```python
from build123d import *

# Parameters (mm, degrees)
F0_W          = 35
F0_H          = 89
F1_DEPTH      = 63
F2_T          = -4
F3_W          = 27
F3_H          = 7.0524177253
F4_DEPTH      = 4.3
F5_DEPTH      = 5.2
F7_DEPTH      = 12
F9_DEPTH      = 28.5
F8_W          = 16.7951798066
F8_H          = 6.5415552817
F10_DEPTH     = 15.6
F8_W_2        = 16.8639151379
F8_H_2        = 7.3436973616
F11_DEPTH     = 29.2
F8_W_3        = 16.7673844844
F8_H_3        = 8.8219475001
F12_DEPTH     = 48.1
F13_W         = 10
F13_H         = 10
F14_DEPTH     = 10
F15_W         = 10
F15_H         = 10
F16_DEPTH     = 10
F19_DEPTH     = 10
F20_DEPTH     = 10
F21_T1_DEPTH  = 97.5
F21_T3_DEPTH  = 27
F21_T8_DEPTH  = 94
F21_T13_DEPTH = 110
F21_T18_DEPTH = 110
F21_T23_DEPTH = 94
F21_T29_DEPTH = 97.5
F21_T35_DEPTH = 39.5
F21_T44_DEPTH = 39.5
F21_T50_DEPTH = 97.5


# Not quite as in the source:
# - a fillet or chamfer that OpenCascade refuses, or shapes differently, is made with other operations: its cross-section is extruded or revolved along the edge and cut away or added


with BuildPart() as f1:
    # F0 (on Top) → F1 (new body)
    with BuildSketch(Plane.XY):
        Rectangle(F0_W, F0_H)
    extrude(amount=F1_DEPTH)

    # F2
    f2_openings = [f1.faces().sort_by_distance(p)[0] for p in [
        (0, 0, 63),
    ]]
    offset(amount=F2_T, openings=f2_openings)

    # F3 (on face) → F4 (cut)
    with BuildSketch(Plane.XY.offset(4)):
        with Locations((0, 36.9737911373)):
            Rectangle(F3_W, F3_H)
    extrude(amount=-F4_DEPTH, mode=Mode.SUBTRACT)

    # F5 (cut): a face of the model
    f5_faces = [f1.faces().sort_by_distance(p)[0] for p in [
        (0, -40.5, 33.5),
    ]]
    extrude(f5_faces, amount=-F5_DEPTH, mode=Mode.SUBTRACT)

    # F7 (add): a face of the model
    f7_faces = [f1.faces().sort_by_distance(p)[0] for p in [
        (-16.5436527827, 0, 63),
    ]]
    extrude(f7_faces, amount=F7_DEPTH)

    # F6 (on face) → F9 (join)
    with BuildSketch(Plane(origin=(13.5, 0, 0), x_dir=(0, -1, 0), z_dir=(-1, 0, 0))):
        Polygon((44.5, 63), (-33.4475822747, 4), (-24.9599814415, 4), (44.5, 56.4169287682), align=None)
    extrude(amount=F9_DEPTH)

    # F8 (on face) → F10 (join)
    with BuildSketch(Plane.XY.offset(4)):
        with Locations((-0.0789728947, 8.664857829)):
            Rectangle(F8_W, F8_H)
    extrude(amount=F10_DEPTH)

    # F8 (on face) → F11 (join)
    with BuildSketch(Plane.XY.offset(4)):
        with Locations((-0.044605229, -10.0223287009)):
            Rectangle(F8_W_2, F8_H_2)
    extrude(amount=F11_DEPTH)

    # F8 (on face) → F12 (join)
    with BuildSketch(Plane.XY.offset(4)):
        with Locations((-0.0928705558, -34.9372858182)):
            Rectangle(F8_W_3, F8_H_3)
    extrude(amount=F12_DEPTH)

    # F13 (on face) → F14 (join)
    with BuildSketch(Plane.YZ.offset(17.5)):
        with Locations((-39.5, 70)):
            Rectangle(F13_W, F13_H)
        with Locations((39.5, 70)):
            Rectangle(F13_W, F13_H)
    extrude(amount=F14_DEPTH)

    # F15 (on face) → F16 (join)
    with BuildSketch(Plane(origin=(-17.5, 0, 0), x_dir=(0, -1, 0), z_dir=(-1, 0, 0))):
        with Locations((-39.5, 70)):
            Rectangle(F15_W, F15_H)
        with Locations((39.5, 70)):
            Rectangle(F15_W, F15_H)
    extrude(amount=F16_DEPTH)

    # F18 (on face) → F19 (cut)
    with BuildSketch(Plane.XZ.offset(44.5)):
        Polygon((-17.5, 65), (-27.5, 75), (-27.5, 65), align=None)
        Polygon((27.5, 75), (17.5, 65), (27.5, 65), align=None)
    extrude(amount=-F19_DEPTH, mode=Mode.SUBTRACT)

    # F17 (on face) → F20 (cut)
    with BuildSketch(Plane(origin=(0, 44.5, 0), x_dir=(-1, 0, 0), z_dir=(0, 1, 0))):
        Polygon((-17.5, 65), (-27.5, 75), (-27.5, 65), align=None)
        Polygon((27.5, 65), (27.5, 75), (17.5, 65), align=None)
    extrude(amount=-F20_DEPTH, mode=Mode.SUBTRACT)

    # F21: fillet of radius 5 on 7 edges, made by hand

    # F21_s2 → F21_t1 (cut)
    with BuildSketch(Plane.XZ.offset(-40.5)):
        with BuildLine():
            ThreePointArc((-18.5, 75), (-14.9644660941, 73.5355339059), (-13.5, 70))
            Line((-13.5, 70), (-13.5, 75))
            Line((-13.5, 75), (-18.5, 75))
        make_face()
        with BuildLine():
            ThreePointArc((18.5, 75), (14.9644660941, 73.5355339059), (13.5, 70))
            Line((13.5, 70), (13.5, 75))
            Line((13.5, 75), (18.5, 75))
        make_face()
    extrude(amount=F21_T1_DEPTH, mode=Mode.SUBTRACT)

    # F21_s4 → F21_t3 (cut)
    with BuildSketch(Plane.YZ.offset(-13.5)):
        with BuildLine():
            ThreePointArc((45.5, 75), (41.9644660941, 73.5355339059), (40.5, 70))
            Line((40.5, 70), (40.5, 75))
            Line((40.5, 75), (45.5, 75))
        make_face()
    extrude(amount=F21_T3_DEPTH, mode=Mode.SUBTRACT)


with BuildPart() as f21_tool6:
    # F21_s7 → F21_t8 (new body)
    with BuildSketch(Plane.XZ.offset(-47)):
        with BuildLine():
            ThreePointArc((-12.5, 75), (-16.0355339059, 73.5355339059), (-17.5, 70))
            Line((-17.5, 70), (-17.5, 75))
            Line((-17.5, 75), (-12.5, 75))
        make_face()
    extrude(amount=F21_T8_DEPTH)

    split(bisect_by=Plane.YZ.offset(-13.5), keep=Keep.TOP)


with BuildPart() as f1_1:
    add(f1.part)

    # F21_t5: cut F21_tool6
    add(f21_tool6.part, mode=Mode.SUBTRACT)


with BuildPart() as f21_tool11:
    # F21_s12 → F21_t13 (new body)
    with BuildSketch(Plane.XZ.offset(57)):
        with BuildLine():
            ThreePointArc((-18.5, 75), (-14.9644660941, 73.5355339059), (-13.5, 70))
            Line((-13.5, 70), (-13.5, 75))
            Line((-13.5, 75), (-18.5, 75))
        make_face()
    extrude(amount=-F21_T13_DEPTH)

    split(bisect_by=Plane.YZ.offset(-17.5), keep=Keep.BOTTOM)


with BuildPart() as f1_2:
    add(f1_1.part)

    # F21_t10: cut F21_tool11
    add(f21_tool11.part, mode=Mode.SUBTRACT)


with BuildPart() as f21_tool16:
    # F21_s17 → F21_t18 (new body)
    with BuildSketch(Plane.XZ.offset(-53)):
        with BuildLine():
            ThreePointArc((18.5, 75), (14.9644660941, 73.5355339059), (13.5, 70))
            Line((13.5, 70), (13.5, 75))
            Line((13.5, 75), (18.5, 75))
        make_face()
    extrude(amount=F21_T18_DEPTH)

    split(bisect_by=Plane.YZ.offset(17.5), keep=Keep.TOP)


with BuildPart() as f1_3:
    add(f1_2.part)

    # F21_t15: cut F21_tool16
    add(f21_tool16.part, mode=Mode.SUBTRACT)


with BuildPart() as f21_tool21:
    # F21_s22 → F21_t23 (new body)
    with BuildSketch(Plane.XZ.offset(47)):
        with BuildLine():
            ThreePointArc((17.5, 70), (16.0355339059, 73.5355339059), (12.5, 75))
            Line((12.5, 75), (17.5, 75))
            Line((17.5, 75), (17.5, 70))
        make_face()
    extrude(amount=-F21_T23_DEPTH)

    split(bisect_by=Plane.YZ.offset(13.5), keep=Keep.BOTTOM)


with BuildPart() as f1_4:
    add(f1_3.part)

    # F21_t20: cut F21_tool21
    add(f21_tool21.part, mode=Mode.SUBTRACT)


with BuildPart() as f21_tool27:
    # F21_s28 → F21_t29 (new body)
    with BuildSketch(Plane.XZ.offset(44.5)):
        with BuildLine():
            ThreePointArc((-18.5, 75), (-14.9644660941, 73.5355339059), (-13.5, 70))
            Line((-13.5, 70), (-13.5, 75))
            Line((-13.5, 75), (-18.5, 75))
        make_face()
    extrude(amount=-F21_T29_DEPTH)

    split(bisect_by=Plane.YZ.offset(-17.5), keep=Keep.TOP)

    split(bisect_by=Plane.XZ.offset(-44.5), keep=Keep.TOP)

    split(bisect_by=Plane.XZ.offset(-40.5), keep=Keep.BOTTOM)


with BuildPart() as f21_tool33:
    # F21_s34 → F21_t35 (new body)
    with BuildSketch(Plane.YZ.offset(13.5)):
        with BuildLine():
            ThreePointArc((45.5, 75), (41.9644660941, 73.5355339059), (40.5, 70))
            Line((40.5, 70), (40.5, 75))
            Line((40.5, 75), (45.5, 75))
        make_face()
    extrude(amount=-F21_T35_DEPTH)

    split(bisect_by=Plane.YZ.offset(-13.5), keep=Keep.BOTTOM)

    split(bisect_by=Plane.XZ.offset(-44.5), keep=Keep.TOP)

    split(bisect_by=Plane(origin=(23.75, 0, 23.75), x_dir=(0, 1, 0), z_dir=(0.7071067812, 0, 0.7071067812)), keep=Keep.TOP)


with BuildPart() as f21_tool27_1:
    add(f21_tool27.part)

    # F21_t39: intersect F21_tool33
    add(f21_tool33.part, mode=Mode.INTERSECT)


with BuildPart() as f1_5:
    add(f1_4.part)

    # F21_t25: cut F21_tool27
    add(f21_tool27_1.part, mode=Mode.SUBTRACT)


with BuildPart() as f21_tool42:
    # F21_s43 → F21_t44 (new body)
    with BuildSketch(Plane.YZ.offset(26)):
        with BuildLine():
            ThreePointArc((45.5, 75), (41.9644660941, 73.5355339059), (40.5, 70))
            Line((40.5, 70), (40.5, 75))
            Line((40.5, 75), (45.5, 75))
        make_face()
    extrude(amount=-F21_T44_DEPTH)

    split(bisect_by=Plane.YZ.offset(13.5), keep=Keep.TOP)

    split(bisect_by=Plane.XZ.offset(-44.5), keep=Keep.TOP)

    split(bisect_by=Plane(origin=(-23.75, 0, 23.75), x_dir=(0, 1, 0), z_dir=(-0.7071067812, 0, 0.7071067812)), keep=Keep.TOP)


with BuildPart() as f21_tool48:
    # F21_s49 → F21_t50 (new body)
    with BuildSketch(Plane.XZ.offset(-53)):
        with BuildLine():
            ThreePointArc((18.5, 75), (14.9644660941, 73.5355339059), (13.5, 70))
            Line((13.5, 70), (13.5, 75))
            Line((13.5, 75), (18.5, 75))
        make_face()
    extrude(amount=F21_T50_DEPTH)

    split(bisect_by=Plane.YZ.offset(17.5), keep=Keep.BOTTOM)

    split(bisect_by=Plane.XZ.offset(-44.5), keep=Keep.TOP)

    split(bisect_by=Plane.XZ.offset(-40.5), keep=Keep.BOTTOM)


with BuildPart() as f21_tool42_1:
    add(f21_tool42.part)

    # F21_t54: intersect F21_tool48
    add(f21_tool48.part, mode=Mode.INTERSECT)


with BuildPart() as f1_6:
    add(f1_5.part)

    # F21_t40: cut F21_tool42
    add(f21_tool42_1.part, mode=Mode.SUBTRACT)


solid = f1_6.part
```
Here's how the part is built. I have some questions about the finished solid (model axes, mm). A direction names the side the tool comes from. Give positions to 0.01 mm unless a question says otherwise; leave off trailing zeros. Loops run counter-clockwise (first coordinate to the right, second up) from the corner with the lowest first, then second, coordinate; pieces in that order, holes last. Notation, with made-up numbers: (-36.5, -13) -> (-23.5, -13) arc R26 ccw to (-23.5, 1) -> close; hole circle Ø11 at (26, -28). An arc over 180 degrees is marked (long way). Use one line per item in the form item = value. Start each with the question number.
1) Imagine slicing it at B-B (z = 26.5). Please give me the cut outline in (x, y), then the cut area to 3 significant figures.
2) Imagine slicing it at A-A (x = -1). Please give me the cut outline in (y, z), then the cut area to 3 significant figures.
3) Imagine slicing it at C-C (x = -20). Please give me the cut outline in (y, z), then the cut area to 3 significant figures.
4) Please list where these lines run through material, in increasing order: line 1 along X through (y, z) = (14, 66.5); line 2 along X through (y, z) = (10.5, 6.5); line 3 along Y through (x, z) = (2, 17).
5) Imagine slicing it at D-D (z = 12.5). Please give me the cut outline in (x, y), then the cut area to 3 significant figures.
6) For P1, Ø13.5, axis at x = -6.5, y = 4, coming from the +Z side; P2, Ø7, axis at y = 8.5, z = 11.5, coming from the -X side; P3, Ø3.5, axis at y = -10.5, z = 24.5, coming from the +X side, each with a flat end and sliding along its axis, tell me the tip position at first contact or that it passes through.
7) Thinking about a two-plate mould opening in Z: for faces 1 (the face through (22.4, 39.6, 69.9)), 2 (the face through (-23, -39, 75)), 3 (the face through (0, -6.35, 16)), 4 (the face through (-8.477, 9, 10)), which applies, +Z half, -Z half, draft (parallel to the pull), parting line (faces both ways), or undercut?
8) Which directions (+Z, -Z, +X, -X, +Y, -Y) give clear straight access to the entire face, cutting with the end or side of a thin tool? Please do faces 5 (the face through (0, -2, 4)), 6 (the face through (20, -34.5, 72)), 7 (the face through (0, -39.348, 28)), 8 (the face through (0, 40.5, 35)), 9 (the face through (-20, 34.5, 72)).
Check values:
q1.outline = (-17.5, -44.5) -> (-13.5, -44.5) -> (-13.5, -4.86) -> (13.5, -4.86) -> (13.5, -44.5) -> (17.5, -44.5) -> (17.5, 44.5) -> (-17.5, 44.5) -> close; (-8.48, -39.35) -> (8.29, -39.35) -> (8.29, -30.53) -> (-8.48, -30.53) -> close; (-8.48, -13.69) -> (8.39, -13.69) -> (8.39, -6.35) -> (-8.48, -6.35) -> close; hole (-13.5, 3.72) -> (13.5, 3.72) -> (13.5, 40.5) -> (-13.5, 40.5) -> close
q1.area = 1,320 mm^2
q2.outline = (-44.5, 0) -> (33.45, 0) -> (33.45, 4) -> (-44.5, 63) -> (-44.5, 56.42) -> (-38.78, 52.1) -> (-39.35, 52.1) -> (-39.35, 4) -> (-44.5, 4) -> close; (40.5, 0) -> (44.5, 0) -> (44.5, 74.9) arc R5 ccw to (40.5, 70) -> close; hole (-30.53, 4) -> (-13.69, 4) -> (-13.69, 33.17) -> (-30.53, 45.87) -> close; hole (-6.35, 4) -> (5.39, 4) -> (5.39, 18.77) -> (-6.35, 27.63) -> close; hole (11.94, 4) -> (24.96, 4) -> (11.94, 13.83) -> close
q2.area = 1,760 mm^2
q3.outline = (-44.5, 67.5) -> (-34.5, 67.5) -> (-34.5, 75) -> (-44.5, 75) -> close; (34.5, 67.5) -> (44.5, 67.5) -> (44.5, 75) -> (34.5, 75) -> close
q3.area = 150 mm^2
q4.line_1 = -17.5 to -13.5, 13.5 to 17.5
q4.line_2 = -17.5 to -13.5, -8.48 to 8.32, 13.5 to 17.5
q4.line_3 = -39.35 to -30.53, -13.69 to -6.35, 5.39 to 16.27, 40.5 to 44.5
q5.outline = (-17.5, -44.5) -> (-13.5, -44.5) -> (-13.5, 13.7) -> (13.5, 13.7) -> (13.5, -44.5) -> (17.5, -44.5) -> (17.5, 44.5) -> (-17.5, 44.5) -> close; (-8.48, -39.35) -> (8.29, -39.35) -> (8.29, -30.53) -> (-8.48, -30.53) -> close; (-8.48, -13.69) -> (8.39, -13.69) -> (8.39, -6.35) -> (-8.48, -6.35) -> close; (-8.48, 5.39) -> (8.32, 5.39) -> (8.32, 11.94) -> (-8.48, 11.94) -> close; hole (-13.5, 22.22) -> (13.5, 22.22) -> (13.5, 40.5) -> (-13.5, 40.5) -> close
q5.area = 1,430 mm^2
q6.P1 = 31.4
q6.P2 = -17.5
q6.P3 = 17.5
q7.face_1 = -Z half
q7.face_2 = +Z half
q7.face_3 = undercut
q7.face_4 = undercut
q8.face_5 = none
q8.face_6 = +Z, -Z, +X
q8.face_7 = -Y
q8.face_8 = +Z, -Z
q8.face_9 = +Z, -Z, -X
